For this review, take the finished solid that the model builds, in its own axes (mm). Coordinates: 2 decimals unless noted, no trailing zeros. Order: outer loops, then holes, each group sorted by start corner. A loop starts at its lowest first (then second) coordinate and runs counter-clockwise, first axis right, second up. Notation, with made-up numbers: (-8, 55.5) -> (16, 55.5) arc R32 cw to (16, 84.5) -> close; hole circle Ø4 at (22, 57). An arc over 180 degrees is marked (long way). Return JSON: item names as keys, results as strings. Group by question number.
Item 1: Take a section at A-A (z = 5.5). Write out the cut boundary in (x, y), then the cut area to 3 significant figures.
Item 2: Insertion check: pin 1 (3 mm diameter, centred on x = -9.5, z = -10.5, fed in from -Y); pin 2 (3.5 mm diameter, centred on y = 7, z = 6, fed in from +X); pin 3 (2 mm diameter, centred on x = 0.5, z = 6, fed in from +Y). Each pin has a flat end and moves straight along its axis. Give the tip position at first contact, or say it passes through.
Item 3: Take a section at C-C (z = 16). Write out the cut boundary in (x, y), then the cut area to 3 significant figures.
Item 4: For line 1 along X through (y, z) = (1.5, 16); line 2 along X through (y, z) = (15.5, -12); line 3 along Y through (x, z) = (18, 15), list the stretches that pass through material, from the lowest coordinate up.
Item 5: Take a section at B-B (y = 6.75). Write out the cut boundary in (x, z), then the cut area to 3 significant figures.
Item 6: Draft analysis for pull direction Y (two halves, no side actions). For faces 1 (the flat face through (-19.56, 14.96, -0.09)), 2 (the flat face through (0, 7, -20)), 3 (the cylindrical face through (21.283, 13.863, 0.496)), state which applies: +Y half, -Y half, draft (parallel to the pull), parting line (faces both ways), or undercut.
```python
from build123d import *

# Parameters (mm, degrees)
SKETCH3_W           = 40
SKETCH3_H           = 40
BOSS_EXTRUDE3_DEPTH = 15
SKETCH5_W           = 53.617813986
SKETCH5_H           = 48.453012442
CUT_EXTRUDE1_DEPTH  = 6
SKETCH6_R           = 20
BOSS_EXTRUDE4_DEPTH = 5


with BuildPart() as part:
    # Sketch3 → Boss-Extrude3 (new body)
    with BuildSketch(Plane(origin=(0, 0, 0), x_dir=(1, 0, 0), z_dir=(0, 1, 0))):
        Rectangle(SKETCH3_W, SKETCH3_H)
    extrude(amount=BOSS_EXTRUDE3_DEPTH)

    # Sketch5 → Cut-Extrude1 (cut)
    with BuildSketch(Plane(origin=(1.150438863, 13.149576371, 0), x_dir=(0, 0, 1), z_dir=(0.08715574274765836, 0.9961946980917455, 0))):
        Rectangle(SKETCH5_W, SKETCH5_H)
    extrude(amount=CUT_EXTRUDE1_DEPTH, mode=Mode.SUBTRACT)

    # Sketch6 → Boss-Extrude4 (add)
    with BuildSketch(Plane(origin=(1.150438863, 13.149576371, 0), x_dir=(0.9961946980917455, -0.08715574274765835, 0), z_dir=(0.08715574274765836, 0.9961946980917457, 0))):
        with Locations(Location((0, 0, 0), (0, 0, 341.098728442))):
            Circle(SKETCH6_R)
    extrude(amount=BOSS_EXTRUDE4_DEPTH)


solid = part.part
```
Findings below:
{
 "1": {"outline": "(-20, 0) -> (20, 0) -> (20, 11.5) -> (20.31, 11.47) -> (20.74, 16.45) -> (-17.57, 19.81) -> (-18.01, 14.83) -> (-20, 15) -> close", "area": "722 mm2"},
 "2": {"pin 1": "stops at y = 0", "pin 2": "stops at x = 20", "pin 3": "stops at y = 18.31"},
 "3": {"outline": "(-20, 0) -> (20, 0) -> (20, 11.5) -> (13.1, 12.1) -> (13.54, 17.08) -> (-10.37, 19.18) -> (-10.8, 14.2) -> (-20, 15) -> close", "area": "650 mm2"},
 "4": {"line 1": "x = -20 to 20", "line 2": "x = -14.71 to 17.42", "line 3": "y = 0 to 11.68"},
 "5": {"outline": "(-20, -20) -> (20, -20) -> (20, 20) -> (-20, 20) -> close", "area": "1,600 mm2"},
 "6": {"face 1": "+Y half", "face 2": "draft", "face 3": "undercut"}
}
